Source: CAD feature listing. Evaluate the final solid. Frame: model axes, mm. Give positions to 0.01 mm unless a question says otherwise; leave off trailing zeros.
Autodesk Inventor part; units mm, degrees
ref_plane "YZ Plane" through (0, 0, 0) normal (1, 0, 0) x (0, 1, 0)
ref_plane "XZ Plane" through (0, 0, 0) normal (0, 1, 0) x (-1, 0, 0)
ref_plane "XY Plane" through (0, 0, 0) normal (0, 0, 1) x (1, 0, 0)
sketch "Skizze1" plane through (-4.3917, 11.7982, 0) normal (0, 0, -1) x (-1, 0, 0)
  circle A0 centre (-0.2488, -4.8451) radius 16.9829
  point P0 (-4.3917, -11.7982)
extrude "Extrusion1" add sketch "Skizze1" along normal blind 4 and the other way blind 2
fillet "Rundung1" radius 2 1 edges at (12.8401, 6.9531, 2)
sketch "Skizze2" plane through (-4.1429, 6.9531, 2) normal (0, 0, 1) x (1, 0, 0)
  circle A0 centre (0, 0) radius 14.9829 construction
  point P0 (4.1429, -6.9531)
  point P1 (0, 11)
  dimension "d5" = 11
hole "Bohrung1" at (-4.1429, 17.9531, 2) direction (0, 0, -1) diameter 2.9 end through all
pattern_circular "Runde Anordnung1" count 8 over 360 about axis through (-4.1429, 6.9531, 0) along (0, 0, -1) of "Bohrung1"
properties part number "Pointing_Finger"
1. Cut plane A-A, the plane z = 0.4. State how many separate pieces and enclosed holes the cut face has, then the cut area to 3 significant figures.
2. Contact query for flat-ended pins moving along their axis: P1, Ø3, axis at x = 3, z = -3, coming from the -Y side; P2, Ø2.5, axis at x = -15.14, y = 6.95, coming from the -Z side; P3, Ø4.5, axis at x = -11.92, y = -0.83, coming from the -Z side; P4, Ø1.5, axis at x = -17.5, z = -1.5, coming from the +Y side. Output: stop coordinate, or through.
3. Line query: L1, parallel to Y at x = 3.5, z = -0.75; L2, parallel to Y at x = -12.5, z = -3.6; L3, parallel to X at y = -2, z = 0.4. Output: solid intervals per line, ascending.
4. Mould query, pull axis X, two halves, no side actions, for faces 1 (the cylindrical face through (2.25, -1.26, -1.04)), 2 (the flat face through (-4, 7, -4)), 3 (the cylindrical face through (-1.93, 23.79, -2.03)). Classes: +X half, -X half, draft (parallel to the pull), parting line (faces both ways), or undercut.
Response values:
1. separate pieces: 1
1. enclosed holes: 8
1. area: 849 mm2
2. P1: stops at y = -9.06
2. P2: passes through
2. P3: stops at z = -4
2. P4: stops at y = 18.33
3. L1: y = -8.21 to -2.27, 0.62 to 13.29, 16.17 to 22.12
3. L2: y = -7.83 to -2.15, 0.5 to 13.4, 16.06 to 21.74
3. L3: x = -18.53 to -12.77, -11.07 to 2.79, 4.49 to 10.24
4. face 1: undercut
4. face 2: draft
4. face 3: parting line
